```python
from build123d import *

# Parameters (mm, degrees)
F0_R     = 21.5
F0_R_2   = 4.1
F1_DEPTH = 2
F2_R     = 11.75
F2_R_2   = 4.1
F3_DEPTH = 9
F4_R     = 10.75
F4_R_2   = 7.25
F5_DEPTH = 3.5
F6_DEPTH = 2.5
F7_R     = 7.25
F7_R_2   = 4.1
F7_R_3   = 3.25
F8_DEPTH = 1


with BuildPart() as f1:
    # F0 (on Top) → F1 (new body)
    with BuildSketch(Plane.XY):
        Circle(F0_R)
        Circle(F0_R_2, mode=Mode.SUBTRACT)
    extrude(amount=F1_DEPTH)

    # F2 (on face) → F3 (join)
    with BuildSketch(Plane.XY.offset(2)):
        Circle(F2_R)
        Circle(F2_R_2, mode=Mode.SUBTRACT)
    extrude(amount=F3_DEPTH)

    # F4 (on face) → F5 (cut)
    with BuildSketch(Plane.XY.offset(11)):
        Circle(F4_R)
        Circle(F4_R_2, mode=Mode.SUBTRACT)
    extrude(amount=-F5_DEPTH, mode=Mode.SUBTRACT)

    # F6 (cut): a face of the model
    f6_faces = [f1.faces().sort_by_distance(p)[0] for p in [
        (-7.0449390335, 0, 11),
    ]]
    extrude(f6_faces, amount=-F6_DEPTH, mode=Mode.SUBTRACT)

    # F7 (on face) → F8 (join)
    with BuildSketch(Plane.XY.offset(8.5)):
        Circle(F7_R)
        Circle(F7_R_2, mode=Mode.SUBTRACT)
        Circle(F7_R_2)
        Circle(F7_R_3, mode=Mode.SUBTRACT)
    extrude(amount=F8_DEPTH)


solid = f1.part
```
The model under review builds one solid part; all positions refer to its coordinate system, in mm. A direction names the side the tool comes from. Round coordinates to 2 decimals unless told otherwise and drop trailing zeros. Loops run counter-clockwise (first coordinate to the right, second up) from the corner with the lowest first, then second, coordinate; pieces in that order, holes last. Notation, with made-up numbers: M 59,-37.75 L 73,-37.75 A29 cw 73,-7.75 Z; hole C 44.25,87 d8. An arc over 180 degrees is marked long. Answer as a JSON object with one key per item and string values.
(1) Take a section at D-D on y = -9.5. Give the boundary of the cut face in (x, z), and give its area (3 significant figures).
Resolved:
{"outline": "M -19.29,0 L 19.29,0 L 19.29,2 L 6.91,2 L 6.91,11 L 5.03,11 L 5.03,7.5 L -5.03,7.5 L -5.03,11 L -6.91,11 L -6.91,2 L -19.29,2 Z", "area": "166 mm²"}
(2) Take a section at A-A on x = 0. Give the boundary of the cut face in (y, z), and give its area (3 significant figures).
Resolved:
{"outline": "M -21.5,0 L -4.1,0 L -4.1,8.5 L -3.25,8.5 L -3.25,9.5 L -7.25,9.5 L -7.25,7.5 L -10.75,7.5 L -10.75,11 L -11.75,11 L -11.75,2 L -21.5,2 Z; M 3.25,8.5 L 4.1,8.5 L 4.1,0 L 21.5,0 L 21.5,2 L 11.75,2 L 11.75,11 L 10.75,11 L 10.75,7.5 L 7.25,7.5 L 7.25,9.5 L 3.25,9.5 Z", "area": "175 mm²"}
(3) Clearance check with flat-ended pins moving along their axes: P1, Ø2.5, axis at x = -0.5, y = -1.5, coming from the -Z side; P2, Ø4, axis at x = 4, z = 7.5, coming from the +Y side; P3, Ø3, axis at y = -12.5, z = 1, coming from the -X side; P4, Ø19.5, axis at x = 0, y = 0, coming from the +Z side. State where each tip first meets the part, or that it passes through.
Resolved:
{"P1": "through", "P2": "y = 11.58", "P3": "x = -18.47", "P4": "z = 9.5"}
(4) Draft analysis for pull direction X (two halves, no side actions). For faces 1 (the flat face through (3, -2, 9.5)), 2 (the flat face through (4.5, 0.3, 0)), 3 (the cylindrical face through (-2.799, 21.317, 0.986)), state which applies: released by +X, released by -X, zero draft, split by the parting line, or undercut.
Resolved:
{"face 1": "undercut", "face 2": "zero draft", "face 3": "split by the parting line"}
(5) To check wall thickness, follow line 1 along Y through (x, z) = (0, 8.95); line 2 along Y through (x, z) = (-3, 8.75); line 3 along Y through (x, z) = (0, 6.5). State the ranges of each line that lie inside material, in increasing order.
Resolved:
{"line 1": "-11.75 to -10.75, -7.25 to -3.25, 3.25 to 7.25, 10.75 to 11.75", "line 2": "-11.36 to -10.32, -6.6 to -1.25, 1.25 to 6.6, 10.32 to 11.36", "line 3": "-11.75 to -4.1, 4.1 to 11.75"}
(6) Tool access review of faces 4 (the flat face through (9, -9, 2)), 5 (the cylindrical face through (-0.534, 4.065, 4.19)), 6 (the cylindrical face through (-2.579, -1.978, 8.993)): name each direction out of +Z, -Z, +X, -X, +Y, -Y from which nothing blocks a thin tool from reaching the whole face with its end or side.
Resolved:
{"face 4": "+Z", "face 5": "-Z", "face 6": "+Z, -Z"}
(7) Take a section at C-C on z = 10.25. Give the boundary of the cut face in (x, y), and give its area (3 significant figures).
Resolved:
{"outline": "C 0,0 d23.5; hole C 0,0 d21.5", "area": "70.7 mm²"}
